Check sheet for the modelled part. Datum: model origin and axes. Units: mm. Face numbers are marked on the shaded views. A direction names the side the tool comes from. Give positions to 0.01 mm unless a question says otherwise; leave off trailing zeros. Write each loop counter-clockwise with the first axis right and the second up, starting at its lowest first coordinate (ties: lowest second). Pieces come first, ordered by that corner, then holes. Notation, with made-up numbers: M 16,38.25 L 62,38.25 A19 ccw 62,57.25 Z; hole C -1,-10.75 d8. An arc over 180 degrees is marked long. Use CSV: the item, a comma, the result in double quotes. Start each with the question number.
1. Scan lines: line 1 (Z direction, x = 6.1, y = 25.5); line 2 (Z direction, x = 12.2, y = 85); line 3 (X direction, y = 39, z = 6). Record each from-to range of solid material in increasing order.
2. Cross-section at A-A, the plane y = 75.5. Enter the section's corners in (x, z), and give its area (3 significant figures).
3. Cross-section at D-D, the plane y = 65.5. Enter the section's corners in (x, z).
4. Cross-section at C-C, the plane x = 12. Enter the section's corners in (y, z).
5. Access from +Z, -Z, +X, -X, +Y, -Y to the whole of each face (thin tool, end or side, straight path). Record for the marked faces 1, 2 and 3.
6. Cross-section at B-B, the plane y = 85. Enter the section's corners in (x, z).
7. Depth check by flat-ended pin: P1, Ø2.5, axis at x = 4.5, z = 3.5, coming from the -Y side; P2, Ø1.5, axis at y = 63, z = 9, coming from the -X side; P3, Ø1.5, axis at y = 17.5, z = 7, coming from the +X side; P4, Ø6, axis at x = 5, y = 16.5, coming from the -Z side. Enter the tip coordinate at first touch or a pass-through.
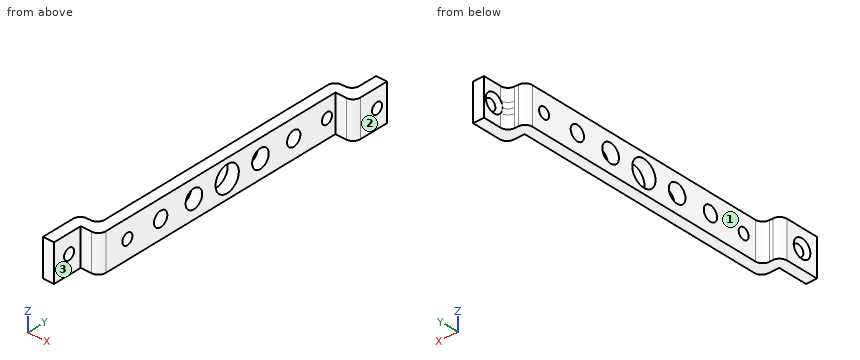
from build123d import *

# Parameters (mm, degrees)
Y_KSEKLIK_EKSTR_ZYON1_DEPTH = 10
IZIM2_W                     = 3
IZIM2_H                     = 10
Y_KSEKLIK_EKSTR_ZYON2_DEPTH = 1
IZIM3_W                     = 3
IZIM3_H                     = 10
Y_KSEKLIK_EKSTR_ZYON3_DEPTH = 1
IZIM4_R                     = 1.5
KES_EKSTR_ZYON1_DEPTH       = 4
PAH1_SIZE                   = 1
IZIM5_R                     = 1.5
KES_EKSTR_ZYON2_DEPTH       = 4
PAH2_SIZE                   = 1
RADYUS1_R                   = 2
IZIM6_R                     = 3.5
IZIM6_R_2                   = 2.5
IZIM6_R_3                   = 2
IZIM6_R_4                   = 1.5
KES_EKSTR_ZYON3_DEPTH       = 4


with BuildPart() as part:
    # Çizim1 → Yükseklik-Ekstrüzyon1 (new body)
    with BuildSketch(Plane.XY):
        Polygon((10, 87), (10, 81), (5, 81), (5, 10), (0, 10), (0, 0), (3, 0), (3, 7), (8, 7), (8, 78), (13, 78), (13, 87), align=None)
    extrude(amount=Y_KSEKLIK_EKSTR_ZYON1_DEPTH)

    # Çizim2 → Yükseklik-Ekstrüzyon2 (add)
    with BuildSketch(Plane(origin=(0, 87, 0), x_dir=(1, 0, 0), z_dir=(0, 1, 0))):
        with Locations((11.5, -5)):
            Rectangle(IZIM2_W, IZIM2_H)
    extrude(amount=Y_KSEKLIK_EKSTR_ZYON2_DEPTH)

    # Çizim3 → Yükseklik-Ekstrüzyon3 (add)
    with BuildSketch(Plane.XZ):
        with Locations((1.5, 5)):
            Rectangle(IZIM3_W, IZIM3_H)
    extrude(amount=Y_KSEKLIK_EKSTR_ZYON3_DEPTH)

    # Çizim4 → Kes-Ekstrüzyon1 (cut)
    with BuildSketch(Plane.ZY.offset(-10)):
        with Locations(Location((5, 85, 0), (0, 0, 270))):
            Circle(IZIM4_R)
    extrude(amount=-KES_EKSTR_ZYON1_DEPTH, mode=Mode.SUBTRACT)

    # Pah1
    pah1_edges = [part.edges().sort_by_distance(p)[0] for p in [
        (10, 86.5, 5),
    ]]
    chamfer(pah1_edges, length=PAH1_SIZE)

    # Çizim5 → Kes-Ekstrüzyon2 (cut)
    with BuildSketch(Plane.ZY):
        with Locations(Location((5, 3.5, 0), (0, 0, 270))):
            Circle(IZIM5_R)
    extrude(amount=-KES_EKSTR_ZYON2_DEPTH, mode=Mode.SUBTRACT)

    # Pah2
    pah2_edges = [part.edges().sort_by_distance(p)[0] for p in [
        (0, 5, 5),
    ]]
    chamfer(pah2_edges, length=PAH2_SIZE)

    # Radyus1
    radyus1_edges = [part.edges().sort_by_distance(p)[0] for p in [
        (13, 78, 5),
        (8, 7, 5),
        (0, 10, 5),
        (5, 10, 5),
        (5, 81, 5),
        (10, 81, 5),
    ]]
    fillet(radyus1_edges, radius=RADYUS1_R)

    # Çizim6 → Kes-Ekstrüzyon3 (cut)
    with BuildSketch(Plane.ZY.offset(-5)):
        with Locations(Location((5, 45.5, 0), (0, 0, 270))):
            Circle(IZIM6_R)
        with Locations(Location((5, 55.5, 0), (0, 0, 270))):
            Circle(IZIM6_R_2)
        with Locations(Location((5, 65.5, 0), (0, 0, 270))):
            Circle(IZIM6_R_3)
        with Locations(Location((5, 75.5, 0), (0, 0, 270))):
            Circle(IZIM6_R_4)
        with Locations(Location((5, 15.5, 0), (0, 0, 270))):
            Circle(IZIM6_R_4)
        with Locations(Location((5, 25.5, 0), (0, 0, 270))):
            Circle(IZIM6_R_3)
        with Locations(Location((5, 35.5, 0), (0, 0, 270))):
            Circle(IZIM6_R_2)
    extrude(amount=-KES_EKSTR_ZYON3_DEPTH, mode=Mode.SUBTRACT)


solid = part.part
Worked answers:
1,line 1,"z = 0 to 3, 7 to 10"
1,line 2,"z = 0 to 3.5, 6.5 to 10"
1,line 3,"x = 5 to 8"
2,outline,"M 5,0 L 8,0 L 8,3.5 L 5,3.5 Z; M 5,6.5 L 8,6.5 L 8,10 L 5,10 Z"
2,area,"21.0 mm^2"
3,outline,"M 5,0 L 8,0 L 8,3 L 5,3 Z; M 5,7 L 8,7 L 8,10 L 5,10 Z"
4,outline,"M 78.27,0 L 88,0 L 88,10 L 78.27,10 Z; hole C 85,5 d3"
5,face 1,"+Z, -Z, -X, +Y"
5,face 2,"+Z, -Z, +X, +Y, -Y"
5,face 3,"+Z, -Z, +X, -Y"
6,outline,"M 10,0 L 13,0 L 13,3.5 L 11,3.5 L 10,2.5 Z; M 10,7.5 L 11,6.5 L 13,6.5 L 13,10 L 10,10 Z"
7,P1,"stops at y = 7"
7,P2,"stops at x = 5"
7,P3,"stops at x = 8"
7,P4,"stops at z = 0"
